Job drawing, mm, ordinate dimensions from the low corner. One solid piece. Give positions to 0.01 mm unless a question says otherwise; leave off trailing zeros. Write each loop counter-clockwise with the first axis right and the second up, starting at its lowest first coordinate (ties: lowest second). Pieces come first, ordered by that corner, then holes. Notation, with made-up numbers: M 70.25,73.25 L 127.25,73.25 A10 cw 127.25,79.25 Z; hole C 47.5,29.25 d1. An arc over 180 degrees is marked long. Use CSV: the item, a comma, the result in double quotes. Start each with the question number.
Item 1: Cut at A-A (z = 24). List the corners of the cut face in (x, y) (1 decimal), then the cut area to 3 significant figures.
Item 2: Cut at B-B (y = 14). List the corners of the cut face in (x, z) (1 decimal), then the cut area to 3 significant figures.
Item 3: Cut at C-C (x = 22). List the corners of the cut face in (y, z), then the cut area to 3 significant figures.
Item 4: Drill centre lines: line 1 (Z direction, x = 28, y = 8.25); line 2 (X direction, y = 18.75, z = 30.5) (1 decimal); line 3 (Z direction, x = 33, y = 24) (1 decimal). Where is each one in solid material? Low to high. Write a range as [from, to].
Item 5: Mould opens along Z. For the marked faces 1, 2 and 3 say: released by +Z, released by -Z, zero draft, split by the parting line, or undercut.
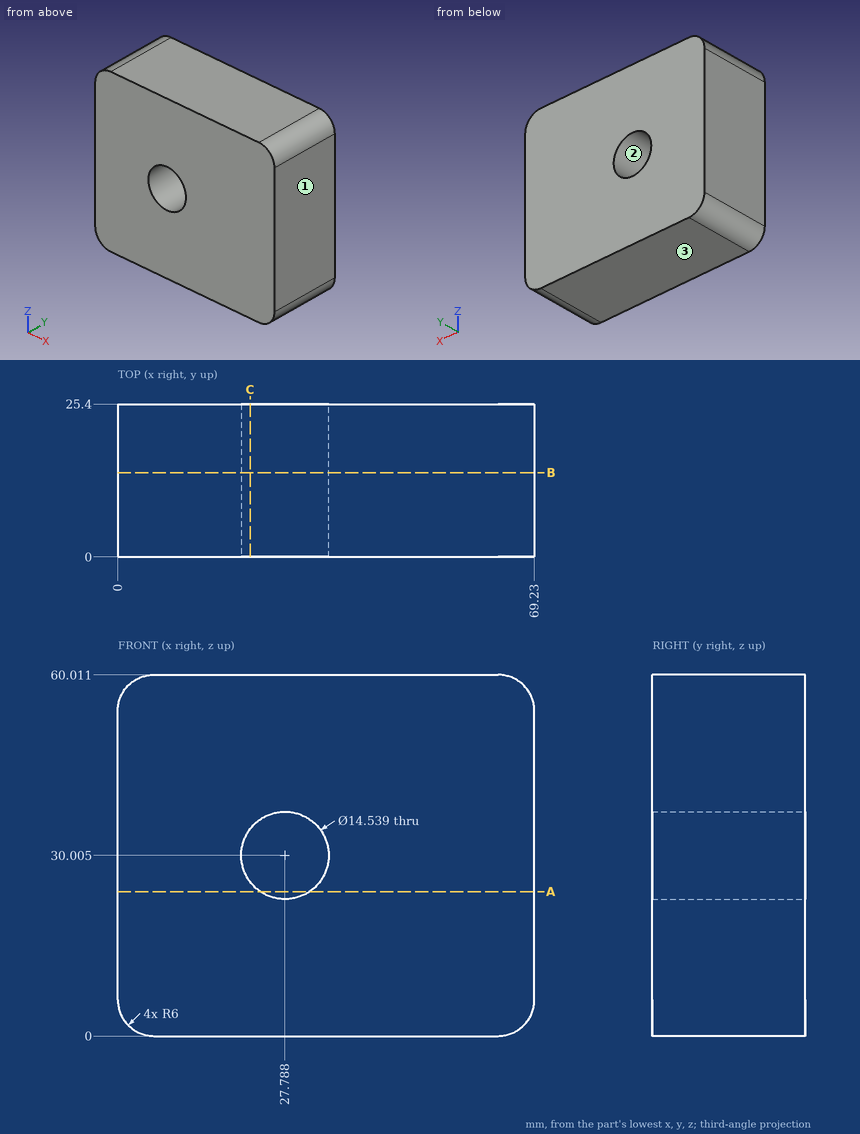
Worked answers:
1,outline,"M 0,0 L 23.7,0 L 23.7,25.4 L 0,25.4 Z; M 31.9,0 L 69.2,0 L 69.2,25.4 L 31.9,25.4 Z"
1,area,"1,550 mm^2"
2,outline,"M 0,6 A6 ccw 6,0 L 63.2,0 A6 ccw 69.2,6 L 69.2,54 A6 ccw 63.2,60 L 6,60 A6 ccw 0,54 Z; hole C 27.8,30 d14.5"
2,area,"3,960 mm^2"
3,outline,"M 0,0 L 25.4,0 L 25.4,25.61 L 0,25.61 Z; M 0,34.4 L 25.4,34.4 L 25.4,60.01 L 0,60.01 Z"
3,area,"1,300 mm^2"
4,line 1,"z = [0, 22.74], [37.27, 60.01]"
4,line 2,"x = [0, 20.5], [35, 69.2]"
4,line 3,"z = [0, 24.9], [35.1, 60]"
5,face 1,"zero draft"
5,face 2,"undercut"
5,face 3,"released by -Z"
